Could you check a few things on this model? Use its own coordinates, in mm. A direction names the side the tool comes from. Give positions to 0.01 mm unless a question says otherwise; leave off trailing zeros. Order: outer loops, then holes, each group sorted by start corner. A loop starts at its lowest first (then second) coordinate and runs counter-clockwise, first axis right, second up. Notation, with made-up numbers: (25.25, 15.5) - (58.25, 15.5) arc R24 ccw to (58.25, 48.5) - close; hole circle Ø2 at (67, 83.5). An arc over 180 degrees is marked (long way). One line per question, with ' | ' between items. Start each with the question number.
1. Which directions (+Z, -Z, +X, -X, +Y, -Y) give clear straight access to the entire face, cutting with the end or side of a thin tool? Please do faces 1 (the flat face through (88, 36, -55.5)), 2 (the cylindrical face through (88.705, -27.935, -53.993)), 3 (the cylindrical face through (-2.343, -17.847, -25.39)), 4 (the cylindrical face through (-3.47, 15.62, -26.14)), 5 (the flat face through (-1, -19, 2)).
2. I need wall thicknesses on probe 1 along Z at (x, y) = (-46, -12.5); probe 2 along Y at (x, z) = (0, -53); probe 3 along Y at (x, z) = (0, -54). Which ranges of each line are inside material? Lowest first, please. Write a range as from..to.
3. Imagine slicing it at C-C (z = -18). Please give me the cut outline in (x, y), and give its area (3 significant figures).
4. If we mould it in two halves opening along Z, with no side actions, what happens to faces 6 (the flat face through (88, -36, 4)), 7 (the cylindrical face through (95.38, -30.04, -52.98)), 8 (the flat face through (-1, -21, 0))? For each: released by +Z, released by -Z, zero draft, split by the parting line, or undercut.
5. For P1, Ø6, axis at x = 21, y = -19.5, coming from the -Z side; P2, Ø1.5, axis at x = -23, y = -38.5, coming from the +Z side; P3, Ø1.5, axis at x = 6, z = -37.5, coming from the +Y side, each with a flat end and sliding along its axis, tell me the tip position at first contact or that it passes through.
```python
from build123d import *

# Parameters (mm, degrees)
F0_R      = 100
F1_DEPTH  = 2
F2_R      = 100
F2_R_2    = 93
F3_DEPTH  = 2
F4_R      = 18
F5_DEPTH  = 51.5
F6_R      = 100
F7_DEPTH  = 2
F8_R      = 100
F8_R_2    = 93
F9_DEPTH  = 2
F10_R     = 1
F11_R     = 16
F12_DEPTH = 69


with BuildPart() as f1:
    # F0 (on Top) → F1 (new body)
    with BuildSketch(Plane.XY):
        Circle(F0_R)
    extrude(amount=F1_DEPTH)

    # F4 (on face) → F5 (join)
    with BuildSketch(Plane(origin=(0, 0, 0), x_dir=(1, 0, 0), z_dir=(0, 0, -1))):
        Circle(F4_R)
    extrude(amount=F5_DEPTH)



with BuildPart() as f3:
    # F2 (on face) → F3 (new body)
    with BuildSketch(Plane(origin=(0, 0, -53.5), x_dir=(1, 0, 0), z_dir=(0, 0, -1))):
        Circle(F2_R)
        Circle(F2_R_2, mode=Mode.SUBTRACT)
    extrude(amount=F3_DEPTH)


with BuildPart() as f1_1:
    add(f1.part)

    add(f3.part)  # F7 merges F3
    # F6 (on face) → F7 (join)
    with BuildSketch(Plane(origin=(0, 0, -51.5), x_dir=(1, 0, 0), z_dir=(0, 0, -1))):
        Circle(F6_R)
    extrude(amount=F7_DEPTH)

    # F8 (on face) → F9 (join)
    with BuildSketch(Plane.XY.offset(2)):
        Circle(F8_R)
        Circle(F8_R_2, mode=Mode.SUBTRACT)
    extrude(amount=F9_DEPTH)

    # F10
    f10_edges = [f1_1.edges().sort_by_distance(p)[0] for p in [
        (-93, 0, -55.5),
        (-100, 0, -55.5),
        (-93, 0, 4),
        (-100, 0, 4),
    ]]
    fillet(f10_edges, radius=F10_R)

    # F11 (on face) → F12 (cut)
    with BuildSketch(Plane(origin=(0, 0, -53.5), x_dir=(1, 0, 0), z_dir=(0, 0, -1))):
        Circle(F11_R)
    extrude(amount=-F12_DEPTH, mode=Mode.SUBTRACT)


solid = f1_1.part
```
Results found:
1) face 1: -Z, +X, -X, +Y, -Y | face 2: -Z | face 3: none | face 4: +Z, -Z | face 5: +Z
2) probe 1: z = -53.5..-51.5, 0..2 | probe 2: y = -100..-16, 16..100 | probe 3: y = -100..-93, 93..100
3) outline: circle Ø36 at (0, 0); hole circle Ø32 at (0, 0) | area: 214 mm2
4) face 6: released by +Z | face 7: zero draft | face 8: undercut
5) P1: stops at z = -53.5 | P2: stops at z = 2 | P3: stops at y = 17.22
